Solid Edge part; units mm, degrees
sketch "Sketch1" plane through (0, 0, 0) normal (0, -1, 0) x (1, 0, 0)
  circle A0 centre (0, 0) radius 12.5
extrude "Protrusion1" add sketch "Sketch1" along normal blind 4
hole "Bohrung_1" at (0, -4, 8) direction (0, 1, 0) diameter 2.2 end through all
pattern_circular "Pattern1" count 8 over 360 about axis through (0, -4, 0) along (0, -1, 0) of "Bohrung_1"
sketch "Sketch2" plane through (0, -4, 0) normal (0, -1, 0) x (1, 0, 0)
  circle A0 centre (0, 0) radius 4.1
extrude "Extrusionsausprägung_2" add sketch "Sketch2" along normal blind 25
hole "Bohrung_2" at (0, -29, 0) direction (0, 1, 0) diameter 3 end through all
hole "Bohrung_3" at (0, 0, 0) direction (0, -1, 0) diameter 8.2 depth 2.3
Verification items for the finished model (mm, model axes). A direction names the side the tool comes from. Coordinates: 2 decimals unless noted, no trailing zeros. Order: outer loops, then holes, each group sorted by start corner. A loop starts at its lowest first (then second) coordinate and runs counter-clockwise, first axis right, second up. Notation, with made-up numbers: (66.25, 29.5) - (87.25, 29.5) arc R28 cw to (87.25, 58.5) - close; hole circle Ø6 at (56, 23.25). An arc over 180 degrees is marked (long way). Return JSON: item names as keys, results as strings.
(1) Access from +Z, -Z, +X, -X, +Y, -Y to the whole of each face (thin tool, end or side, straight path). Record for faces 1 (the cylindrical face through (-0.534, -16.325, -4.065)), 2 (the cylindrical face through (0.421, -2.028, -6.984)), 3 (the flat face through (2, -2.3, 0)).
Filled sheet:
{"face 1": "-Y", "face 2": "+Y, -Y", "face 3": "+Y"}
(2) Section check D-D, the plane y = -26.75. Record the cut outline in (x, z).
Filled sheet:
{"outline": "circle Ø8.2 at (0, 0); hole circle Ø3 at (0, 0)"}
(3) Mould release check, pull along X, two halves, no side actions. Record for faces 4 (the cylindrical face through (6.984, -2.028, 0.421)), 5 (the cylindrical face through (-5.066, -2.028, -6.585)), 6 (the flat face through (-5, 0, 0)), 7 (the cylindrical face through (11.923, -1.972, -3.755)): pulls with the +X half, pulls with the -X half, needs draft (parallel to the pull), parting line crosses it, or undercut.
Filled sheet:
{"face 4": "undercut", "face 5": "undercut", "face 6": "needs draft", "face 7": "parting line crosses it"}
(4) Section check A-A, the plane x = 0. Record the cut outline in (y, z), and give its area (3 significant figures).
Filled sheet:
{"outline": "(-29, -4.1) - (-4, -4.1) - (-4, -6.9) - (0, -6.9) - (0, -4.1) - (-2.3, -4.1) - (-2.3, -1.5) - (-29, -1.5) - close; (-29, 1.5) - (-2.3, 1.5) - (-2.3, 4.1) - (0, 4.1) - (0, 6.9) - (-4, 6.9) - (-4, 4.1) - (-29, 4.1) - close; (-4, -12.5) - (0, -12.5) - (0, -9.1) - (-4, -9.1) - close; (-4, 9.1) - (0, 9.1) - (0, 12.5) - (-4, 12.5) - close", "area": "188 mm^2"}
(5) Section check B-B, the plane z = 8. Record the cut outline in (x, y).
Filled sheet:
{"outline": "(-9.6, -4) - (-1.1, -4) - (-1.1, 0) - (-9.6, 0) - close; (1.1, -4) - (9.6, -4) - (9.6, 0) - (1.1, 0) - close"}
(6) Go/stop test with flat-tipped pins: pin 1 (3 mm diameter, centred on x = -8, z = 0, fed in from -Y); pin 2 (4 mm diameter, centred on x = 2, z = 0, fed in from +Y); pin 3 (6 mm diameter, centred on x = 2.5, y = -12.5, fed in from -Z). Record where each tip stops, or that it passes through.
Filled sheet:
{"pin 1": "stops at y = -4", "pin 2": "stops at y = -2.3", "pin 3": "stops at z = -4.1"}
(7) Thickness scan on line 1 along Z through (x, y) = (0, -0.5); line 2 along Y through (x, z) = (-2.75, 5.25); line 3 along Z through (x, y) = (-8.5, -1). Record the ranges inside material, lowest first.
Filled sheet:
{"line 1": "z = -12.5 to -9.1, -6.9 to -4.1, 4.1 to 6.9, 9.1 to 12.5", "line 2": "y = -4 to 0", "line 3": "z = -9.17 to -0.98, 0.98 to 9.17"}
(8) Section check C-C, the plane x = -6. Record the cut outline in (y, z).
Filled sheet:
{"outline": "(-4, -10.97) - (0, -10.97) - (0, -6.7) - (-4, -6.7) - close; (-4, -4.61) - (0, -4.61) - (0, 4.61) - (-4, 4.61) - close; (-4, 6.7) - (0, 6.7) - (0, 10.97) - (-4, 10.97) - close"}
